Geometry check sheet. Reference: the model listing, model coordinates, mm. Coordinates: 2 decimals unless noted, no trailing zeros. Write each loop counter-clockwise with the first axis right and the second up, starting at its lowest first coordinate (ties: lowest second). Pieces come first, ordered by that corner, then holes. Notation, with made-up numbers: (78, 62.5) -> (113, 62.5) arc R34 cw to (113, 101.5) -> close; hole circle Ø4 at (29, 66.5). An arc over 180 degrees is marked (long way). Put each result on its own line as item: value. Start each with the question number.
Autodesk Inventor part; units mm, degrees
ref_plane "YZ Plane" through (0, 0, 0) normal (1, 0, 0) x (0, 1, 0)
ref_plane "XZ Plane" through (0, 0, 0) normal (0, 1, 0) x (-1, 0, 0)
ref_plane "XY Plane" through (0, 0, 0) normal (0, 0, 1) x (1, 0, 0)
sketch "Sketch1" plane through (0, 0, 0) normal (1, 0, 0) x (0, 1, 0)
  ellipse E0 centre (0, 0) end of major axis (0, -2) minor radius 1.9928
  line L0 (-20.007, -58.0002) -> (-20.007, -89.2502)
  line L1 (-20.007, -89.2502) -> (-25.007, -89.2502)
  line L2 (-25.007, -58.0002) -> (-25.007, -89.2502)
  line L3 (-20.007, -58.0002) -> (-25.007, -58.0002)
  line L4 (-20.007, 31.2498) -> (-20.007, -31.7502)
  line L5 (-20.007, -31.7502) -> (-25.007, -31.7502)
  line L6 (-25.007, 31.2498) -> (-25.007, -31.7502)
  line L7 (-20.007, 31.2498) -> (-25.007, 31.2498)
  line L8 (-20.007, 88.7498) -> (-20.007, 57.4998)
  line L9 (-20.007, 57.4998) -> (-25.007, 57.4998)
  line L10 (-25.007, 88.7498) -> (-25.007, 57.4998)
  line L11 (-20.007, 88.7498) -> (-25.007, 88.7498)
  line L12 (-25.0077, 93.7498) -> (-25.0077, 98.7498)
  line L13 (-10.0085, 98.7498) -> (-25.0077, 98.7498)
  line L14 (-10.0085, 93.7498) -> (-10.0085, 98.7498)
  line L15 (9.9915, 93.7498) -> (9.9915, 98.7498)
  line L16 (19.993, 98.7498) -> (9.9915, 98.7498)
  line L17 (9.9915, 93.7498) -> (-10.0085, 93.7498)
  line L18 (-25.0077, 93.7498) -> (-33.0079, 93.7498)
  line L19 (22.993, -99.2777) -> (9.993, -99.2502)
  line L20 (9.993, -99.2502) -> (9.993, -94.2502)
  line L21 (9.993, -94.2502) -> (-10.0077, -94.2502)
  line L22 (-10.0077, -99.2502) -> (-10.0077, -94.2502)
  line L23 (-10.0077, -99.2502) -> (-25.0077, -99.2502)
  line L24 (-25.0077, -99.2502) -> (-25.0077, -94.2502)
  line L25 (-25.0077, -94.2502) -> (-33.0079, -94.2502)
  line L26 (-33.0079, -94.2502) -> (-33.0079, 93.7498)
  line L27 (22.993, -99.2777) -> (22.993, -94.2502)
  line L28 (22.993, -89.2502) -> (22.993, -94.2502)
  line L29 (22.993, -89.2502) -> (19.993, -89.2502)
  line L30 (19.993, -58.0002) -> (19.993, -89.2502)
  line L31 (22.993, -58.0002) -> (19.993, -58.0002)
  line L32 (22.993, -31.7502) -> (22.993, -58.0002)
  line L33 (22.993, -31.7502) -> (19.993, -31.7502)
  line L34 (19.993, 31.2498) -> (19.993, -31.7502)
  line L35 (22.993, 31.2498) -> (19.993, 31.2498)
  line L36 (22.993, 57.4998) -> (22.993, 31.2498)
  line L37 (22.993, 57.4998) -> (19.993, 57.4998)
  line L38 (19.993, 88.7498) -> (19.993, 57.4998)
  line L39 (22.993, 88.7498) -> (19.993, 88.7498)
  line L40 (22.993, 93.7498) -> (22.993, 88.7498)
  line L41 (22.993, 93.7498) -> (19.993, 93.7498)
  line L42 (19.993, 93.7498) -> (19.993, 98.7498)
  point P0 (-29.9123, 87.1698)
  dimension "d21" = 188
  dimension "d26" = 3
extrude "Extrusion1" add sketch "Sketch1" along normal blind 5
properties part number "case top sides" material "ABS Plastic"
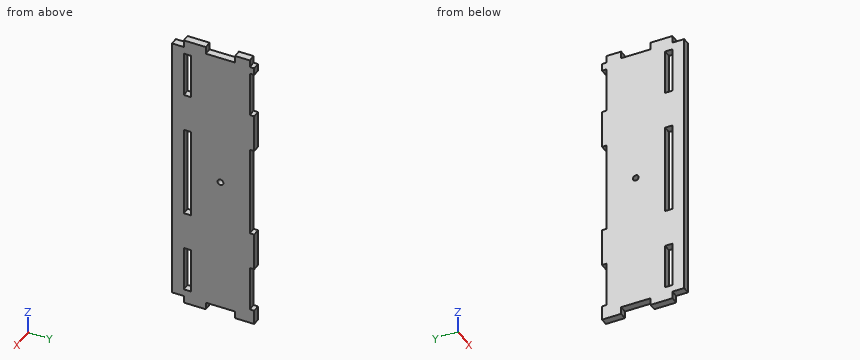
Item 1: Section check B-B, the plane x = 1.55. Give the number of separate pieces and of enclosed holes in the cut face, and give its area (3 significant figures).
Item 2: Section check C-C, the plane y = -7.5. Enter the section's corners in (x, z), and give its area (3 significant figures).
Item 3: Section check A-A, the plane z = -29. Enter the section's corners in (x, y).
Item 4: Go/stop test with flat-tipped pins: P1, Ø2.5, axis at x = 2.5, z = -97, coming from the -Y side; P2, Ø1, axis at x = 4.5, y = 3, coming from the +Z side; P3, Ø2.5, axis at x = 3.5, z = 95.5, coming from the +Y side. Record where each tip stops, or that it passes through.
Item 5: Scan lines: line 1 along Z through (x, y) = (3.45, -21); line 2 along Y through (x, z) = (0.9, 7); line 3 along Z through (x, y) = (3.9, 13). Record each from-to range of solid material in increasing order. Write a range as [from, to].
From the geometry:
1. separate pieces: 1
1. enclosed holes: 4
1. area: 9,780 mm²
2. outline: (0, -94.25) -> (5, -94.25) -> (5, 93.75) -> (0, 93.75) -> close
2. area: 940 mm²
3. outline: (0, -33.01) -> (5, -33.01) -> (5, -25.01) -> (0, -25.01) -> close; (0, -20.01) -> (5, -20.01) -> (5, 19.99) -> (0, 19.99) -> close
4. P1: y = -25.01
4. P2: z = 93.75
4. P3: y = 19.99
5. line 1: [-99.25, -89.25], [-58, -31.75], [31.25, 57.5], [88.75, 98.75]
5. line 2: [-33.01, -25.01], [-20.01, 19.99]
5. line 3: [-99.26, 98.75]
